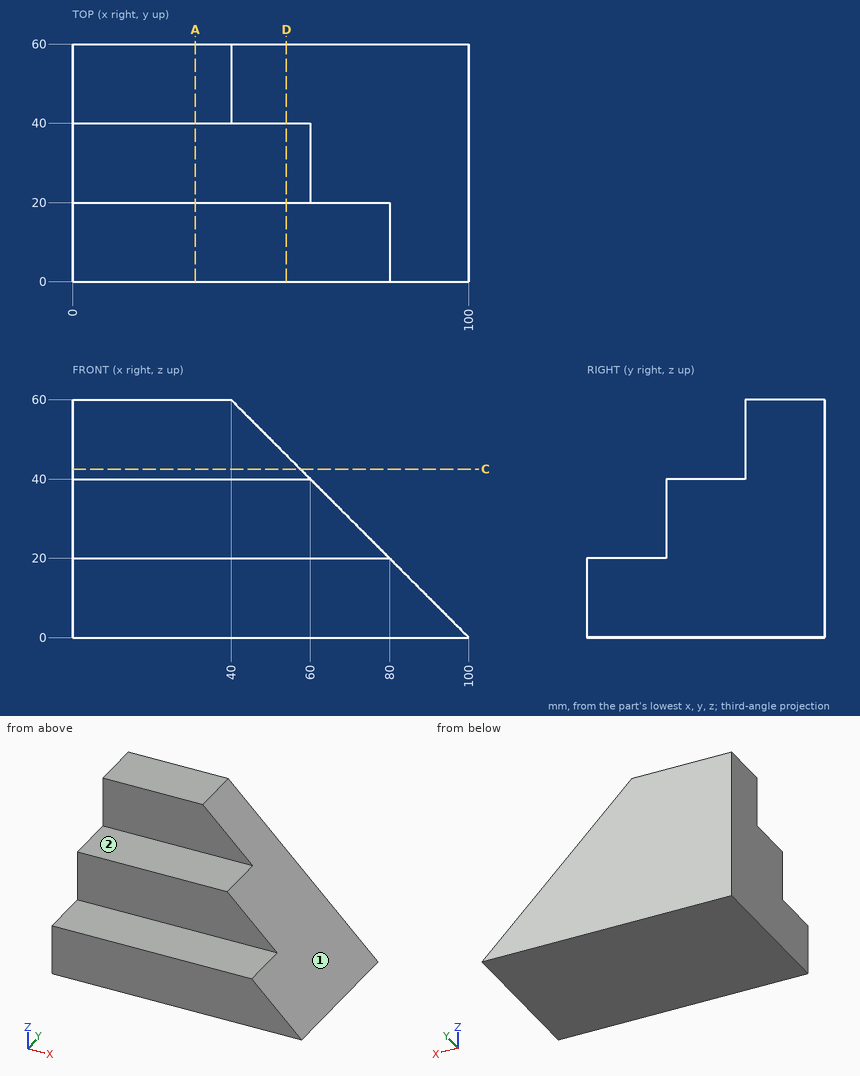
For this review, use the dimensioned drawing (mm, ordinates from the lowest corner) and the shaded views. A direction names the side the tool comes from. Give positions to 0.01 mm unless a question says otherwise; leave off trailing zeros. Write each loop counter-clockwise with the first axis right and the second up, starting at its lowest first coordinate (ties: lowest second). Pieces come first, ordered by that corner, then holes. Notation, with made-up numbers: M -28,0.5 L -1,0.5 A9 cw -1,9.5 Z; hole C 5,43 d1. An arc over 180 degrees is marked long. Answer as a JSON object with one key per item and string values. Group by question number.
Item 1: For probe 1 along Y at (x, z) = (52, 26); probe 2 along Z at (x, y) = (40.5, 11); probe 3 along X at (y, z) = (45, 18), list the stretches that pass through material, from the lowest coordinate up. Write a range as [from, to].
Item 2: Consider section C-C on z = 42.5. Write out the cut boundary in (x, y).
Item 3: Consider section A-A on x = 31. Write out the cut boundary in (y, z).
Item 4: For pin 1 Ø10 at (x, y) = (23, 6) entering from +Z; pin 2 Ø5 at (y, z) = (22.5, 22) entering from +X; pin 3 Ø6 at (x, z) = (33, 29.5) entering from -Y, all flat-tipped, find the tip position at first contact; note any pin that passes through.
Item 5: Consider section D-D on x = 54. Write out the cut boundary in (y, z).
Item 6: Tool access review of the marked faces 1 and 2: name each direction out of +Z, -Z, +X, -X, +Y, -Y from which nothing blocks a thin tool from reaching the whole face with its end or side.
Check result:
{
 "1": {"probe 1": "y = [20, 60]", "probe 2": "z = [0, 20]", "probe 3": "x = [0, 82]"},
 "2": {"outline": "M 0,40 L 57.5,40 L 57.5,60 L 0,60 Z"},
 "3": {"outline": "M 0,0 L 60,0 L 60,60 L 40,60 L 40,40 L 20,40 L 20,20 L 0,20 Z"},
 "4": {"pin 1": "stops at z = 20", "pin 2": "stops at x = 80.5", "pin 3": "stops at y = 20"},
 "5": {"outline": "M 0,0 L 60,0 L 60,46 L 40,46 L 40,40 L 20,40 L 20,20 L 0,20 Z"},
 "6": {"face 1": "+Z, +X, +Y, -Y", "face 2": "+Z, +X, -X, -Y"}
}
